Read the model definition and answer for the solid it produces. Units are mm, in the model's axes. Face numbers are marked on the shaded views. A direction names the side the tool comes from. Coordinates: 2 decimals unless noted, no trailing zeros. Loops run counter-clockwise (first coordinate to the right, second up) from the corner with the lowest first, then second, coordinate; pieces in that order, holes last. Notation, with made-up numbers: (39.25, -38) - (96.25, -38) arc R6 cw to (96.25, -33) - close; hole circle Ø1 at (22, 3). An arc over 180 degrees is marked (long way). Use CSV: the item, a comma, the result in double quotes.
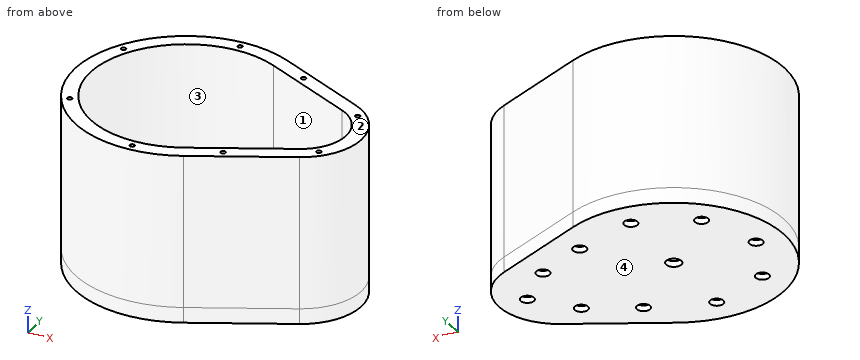
```python
from build123d import *
from build123d.topology import SkipClean

# Parameters (mm, degrees)
SKETCH1_R           = 4
BOSS_EXTRUDE2_DEPTH = 8
BOSS_EXTRUDE3_DEPTH = 16
SKETCH6_R           = 1.55
CUT_EXTRUDE1_DEPTH  = 24
SKETCH7_R           = 8.2
CUT_EXTRUDE2_DEPTH  = 5
SKETCH8_R           = 2
BOSS_EXTRUDE4_DEPTH = 8.5
SKETCH9_R           = 3.5
CUT_EXTRUDE3_DEPTH  = 3
BOSS_EXTRUDE5_DEPTH = 80
SKETCH11_R          = 1.25
CUT_EXTRUDE4_DEPTH  = 10


with BuildPart() as part:
    # Sketch1 → Boss-Extrude2 (new body)
    with BuildSketch(Plane.XY):
        with BuildLine():
            Line((73.9125, 28.261145478), (25.616666667, 52.036394849))
            ThreePointArc((25.616666667, 52.036394849), (-58, 0), (25.616666667, -52.036394849))
            Line((25.616666667, -52.036394849), (73.9125, -28.261145478))
            ThreePointArc((73.9125, -28.261145478), (91.5, 0), (73.9125, 28.261145478))
        make_face()
        Circle(SKETCH1_R, mode=Mode.SUBTRACT)
    extrude(amount=BOSS_EXTRUDE2_DEPTH)

    # Sketch5 → Boss-Extrude3 (add)
    with BuildSketch(Plane.XY.offset(8)):
        with BuildLine():
            Line((20.758333333, 42.167423412), (69.054166667, 18.392174041))
            ThreePointArc((69.054166667, 18.392174041), (80.5, 0), (69.054166667, -18.392174041))
            Line((69.054166667, -18.392174041), (20.758333333, -42.167423412))
            ThreePointArc((20.758333333, -42.167423412), (-47, 0), (20.758333333, 42.167423412))
        make_face()
        with BuildLine():
            Line((65.520833333, 11.214740269), (17.225, 34.98998964))
            ThreePointArc((17.225, 34.98998964), (-39, 0), (17.225, -34.98998964))
            Line((17.225, -34.98998964), (65.520833333, -11.214740269))
            ThreePointArc((65.520833333, -11.214740269), (72.5, 0), (65.520833333, 11.214740269))
        make_face(mode=Mode.SUBTRACT)
    extrude(amount=BOSS_EXTRUDE3_DEPTH)

    # Sketch6 → Cut-Extrude1 (cut)
    with BuildSketch(Plane.XY.offset(24)):
        with Locations((0, 43)):
            Circle(SKETCH6_R)
        with Locations((-30.405591591, 30.405591591)):
            Circle(SKETCH6_R)
        with Locations((-43, 0)):
            Circle(SKETCH6_R)
        with Locations((-30.405591591, -30.405591591)):
            Circle(SKETCH6_R)
        with Locations((0, -43)):
            Circle(SKETCH6_R)
        with Locations((76.5, 0)):
            Circle(SKETCH6_R)
        with Locations((58.315707785, 19.220123822)):
            Circle(SKETCH6_R)
        with Locations((32.44935499, 31.953706526)):
            Circle(SKETCH6_R)
        with Locations((58.315707785, -19.220123822)):
            Circle(SKETCH6_R)
        with Locations((32.44935499, -31.953706526)):
            Circle(SKETCH6_R)
    extrude(amount=-CUT_EXTRUDE1_DEPTH, mode=Mode.SUBTRACT)

    # Sketch7 → Cut-Extrude2 (cut)
    with BuildSketch(Plane.XY.offset(8)):
        Circle(SKETCH7_R)
    extrude(amount=-CUT_EXTRUDE2_DEPTH, mode=Mode.SUBTRACT)

    # Sketch8 → Boss-Extrude4 (add)
    with BuildSketch(Plane.XY.offset(8)):
        with Locations(Location((60, 0, 0), (0, 0, 180))):
            Circle(SKETCH8_R)
    extrude(amount=BOSS_EXTRUDE4_DEPTH)

    # Sketch9 → Cut-Extrude3 (cut)
    with BuildSketch(Plane(origin=(0, 0, 0), x_dir=(-1, 0, 0), z_dir=(0, 0, -1))):
        with Locations((0, 43)):
            Circle(SKETCH9_R)
        with Locations((30.405591591, 30.405591591)):
            Circle(SKETCH9_R)
        with Locations((43, 0)):
            Circle(SKETCH9_R)
        with Locations((30.405591591, -30.405591591)):
            Circle(SKETCH9_R)
        with Locations((0, -43)):
            Circle(SKETCH9_R)
        with Locations((-32.44935499, 31.953706526)):
            Circle(SKETCH9_R)
        with Locations((-32.44935499, -31.953706526)):
            Circle(SKETCH9_R)
        with Locations((-58.315707785, -19.220123822)):
            Circle(SKETCH9_R)
        with Locations((-58.315707785, 19.220123822)):
            Circle(SKETCH9_R)
        with Locations((-76.5, 0)):
            Circle(SKETCH9_R)
    extrude(amount=-CUT_EXTRUDE3_DEPTH, mode=Mode.SUBTRACT)

    # Sketch10 → Boss-Extrude5 (add)
    with SkipClean():  # the faces are left unmerged after this step: merging them gives an invalid solid
        with BuildSketch(Plane.XY.offset(8)):
            with BuildLine():
                Line((25.616666667, 52.036394849), (73.9125, 28.261145478))
                ThreePointArc((73.9125, 28.261145478), (91.5, 0), (73.9125, -28.261145478))
                Line((73.9125, -28.261145478), (25.616666667, -52.036394849))
                ThreePointArc((25.616666667, -52.036394849), (-58, 0), (25.616666667, 52.036394849))
            make_face()
            with BuildLine():
                Line((22.083333333, 44.858961077), (70.379166667, 21.083711706))
                ThreePointArc((70.379166667, 21.083711706), (83.5, 0), (70.379166667, -21.083711706))
                Line((70.379166667, -21.083711706), (22.083333333, -44.858961077))
                ThreePointArc((22.083333333, -44.858961077), (-50, 0), (22.083333333, 44.858961077))
            make_face(mode=Mode.SUBTRACT)
        extrude(amount=BOSS_EXTRUDE5_DEPTH)

    # Sketch11 → Cut-Extrude4 (cut)
    with SkipClean():  # the faces are left unmerged after this step: merging them gives an invalid solid
        with BuildSketch(Plane.XY.offset(88)):
            with Locations((0, 54)):
                Circle(SKETCH11_R)
            with Locations((-46.765371804, 27)):
                Circle(SKETCH11_R)
            with Locations((-46.765371804, -27)):
                Circle(SKETCH11_R)
            with Locations((0, -54)):
                Circle(SKETCH11_R)
            with Locations((40.333245578, 40.333245578)):
                Circle(SKETCH11_R)
            with Locations((40.333245578, -40.333245578)):
                Circle(SKETCH11_R)
            with Locations((79.445436483, 19.445436483)):
                Circle(SKETCH11_R)
            with Locations((79.445436483, -19.445436483)):
                Circle(SKETCH11_R)
        extrude(amount=-CUT_EXTRUDE4_DEPTH, mode=Mode.SUBTRACT)


solid = part.part
```
Q1. The part is cut by section C-C on y = 6. Determine the outline of the cut face in (x, z).
Reported:
outline,"(-57.69, 0) - (90.92, 0) - (90.92, 88) - (82.72, 88) - (82.72, 8) - (79.6, 8) - (79.6, 24) - (70.97, 24) - (70.97, 8) - (5.59, 8) - (5.59, 3) - (-5.59, 3) - (-5.59, 8) - (-38.54, 8) - (-38.54, 24) - (-46.62, 24) - (-46.62, 8) - (-49.64, 8) - (-49.64, 88) - (-57.69, 88) - close"
Q2. Find the intervals of material crossed by probe 1 along Y at (x, z) = (0, 83); probe 2 along X at (y, z) = (40, 14); probe 3 along Y at (x, z) = (-43, 19.25), in increasing order. Write a range as [from, to].
Reported:
probe 1,"y = [-58, -55.25], [-52.75, -50], [50, 52.75], [55.25, 58]"
probe 2,"x = [-42, -30], [-24.68, 25.16], [31.95, 50.07]"
probe 3,"y = [-38.92, -25.51], [-18.97, -1.55], [1.55, 18.97], [25.51, 38.92]"
Q3. A tool of negligible diameter and unlimited length cuts with its end or side. For the marked faces 3 and 4, from which of +Z, -Z, +X, -X, +Y, -Y can it reach the whole face along a straight path? Write none if from no direction.
Reported:
face 3,"+Z"
face 4,"-Z, +X, -X, +Y, -Y"
Q4. Given P1, Ø3.5, axis at x = -0.5, y = 42, coming from the -Z side; P2, Ø1.5, axis at x = 3, y = -7.5, coming from the +Z side; P3, Ø3, axis at x = -4.5, z = 49.5, coming from the -Y side; P4, Ø3, axis at x = 58.32, y = 19.22, coming from the +Z side, each flat-ended and moving along its own axis, determine where each tip first touches the part or whether it passes through.
Reported:
P1,"stops at z = 3"
P2,"stops at z = 8"
P3,"stops at y = -57.92"
P4,"passes through"
Q5. The part is cut by section D-D on x = -13.5. Determine the outline of the cut face in (y, z), and give its area (3 significant figures).
Reported:
outline,"(-56.41, 0) - (56.41, 0) - (56.41, 88) - (48.14, 88) - (48.14, 8) - (45.02, 8) - (45.02, 24) - (36.59, 24) - (36.59, 8) - (-36.59, 8) - (-36.59, 24) - (-45.02, 24) - (-45.02, 8) - (-48.14, 8) - (-48.14, 88) - (-56.41, 88) - close"
area,"2,490 mm²"
Q6. For a pull along X with two mould halves and no side action, classify the marked faces 1 and 2 as +X half, -X half, draft (parallel to the pull), parting line (faces both ways), or undercut.
Reported:
face 1,"undercut"
face 2,"draft"
Q7. The part is cut by section B-B on z = 12. Give the number of separate pieces and of enclosed holes in the cut face, and give its area (3 significant figures).
Reported:
separate pieces,"3"
enclosed holes,"12"
area,"5,590 mm²"
Q8. The part is cut by section A-A on z = 28.5. Determine the outline of the cut face in (x, y).
Reported:
outline,"(25.62, -52.04) - (73.91, -28.26) arc R31.5 ccw to (73.91, 28.26) - (25.62, 52.04) arc R58 ccw (long way) to start; hole (22.08, -44.86) - (70.38, -21.08) arc R23.5 ccw to (70.38, 21.08) - (22.08, 44.86) arc R50 ccw (long way) to start"
